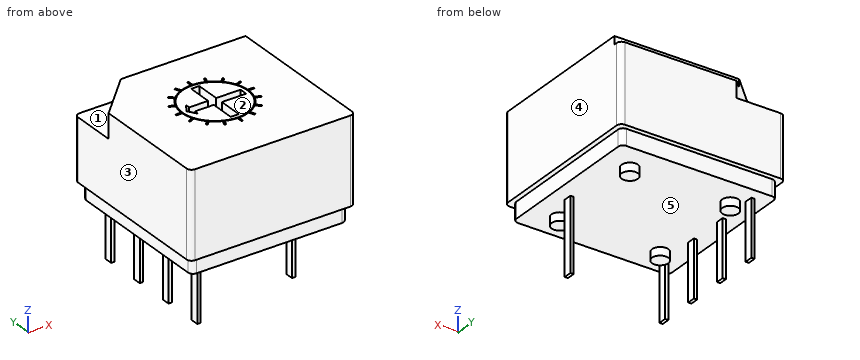
```python
from build123d import *

# Parameters (mm, degrees)
SKETCH1_W               = 10.2
SKETCH1_H               = 10.2
BOSS_EXTRUDE2_DEPTH     = 6.5
SKETCH3_R               = 0.501534086
BOSS_EXTRUDE3_DEPTH     = 0.5
FILLET1_R               = 0.3
SKETCH4_W               = 10.2
SKETCH4_H               = 10.2
SKETCH4_W_2             = 9.6
SKETCH4_H_2             = 9.6
CUT_EXTRUDE_THIN1_DEPTH = 1
FILLET2_R               = 0.3
SKETCH5_W               = 0.2
SKETCH5_H               = 0.5
BOSS_EXTRUDE5_DEPTH     = 3.5
SKETCH6_W               = 0.2
SKETCH6_H               = 0.5
BOSS_EXTRUDE6_DEPTH     = 1
SKETCH7_W               = 10.2
SKETCH7_H               = 10.2
CUT_EXTRUDE3_DEPTH      = 0.2
CUT_EXTRUDE4_DEPTH      = 1.5
CUT_EXTRUDE5_DEPTH      = 0.5
SKETCH10_R              = 2.05
SKETCH10_R_2            = 2
CUT_EXTRUDE6_DEPTH      = 0.5
CUT_EXTRUDE7_DEPTH      = 1
CUT_EXTRUDE8_DEPTH      = 0.3


with BuildPart() as part:
    # Sketch1 → Boss-Extrude2 (new body)
    with BuildSketch(Plane.XY):
        with Locations((5.1, 5.1)):
            Rectangle(SKETCH1_W, SKETCH1_H)
    extrude(amount=BOSS_EXTRUDE2_DEPTH)

    # Sketch3 → Boss-Extrude3 (add)
    with BuildSketch(Plane(origin=(0, 0, 0), x_dir=(-1, 0, 0), z_dir=(0, 0, -1))):
        with Locations((-8.2, 8.2)):
            Circle(SKETCH3_R)
        with Locations(Location((-2, 8.2, 0), (0, 0, 180))):
            Circle(SKETCH3_R)
        with Locations(Location((-8.2, 2, 0), (0, 0, 180))):
            Circle(SKETCH3_R)
        with Locations((-2, 2)):
            Circle(SKETCH3_R)
    extrude(amount=BOSS_EXTRUDE3_DEPTH)

    # Fillet1
    fillet1_edges = [part.edges().sort_by_distance(p)[0] for p in [
        (0, 10.2, 3.25),
        (10.2, 10.2, 3.25),
        (10.2, 0, 3.25),
        (0, 0, 3.25),
    ]]
    fillet(fillet1_edges, radius=FILLET1_R)

    # Sketch4 → Cut-Extrude-Thin1 (cut)
    with BuildSketch(Plane(origin=(0, 0, 0), x_dir=(-1, 0, 0), z_dir=(0, 0, -1))):
        with Locations((-5.1, 5.1)):
            Rectangle(SKETCH4_W, SKETCH4_H)
        with Locations((-5.1, 5.1)):
            Rectangle(SKETCH4_W_2, SKETCH4_H_2, mode=Mode.SUBTRACT)
    extrude(amount=-CUT_EXTRUDE_THIN1_DEPTH, mode=Mode.SUBTRACT)

    # Fillet2
    fillet2_edges = [part.edges().sort_by_distance(p)[0] for p in [
        (9.9, 0.3, 0.5),
        (9.9, 9.9, 0.5),
        (0.3, 9.9, 0.5),
        (0.3, 0.3, 0.5),
    ]]
    fillet(fillet2_edges, radius=FILLET2_R)

    # Sketch5 → Boss-Extrude5 (add)
    with BuildSketch(Plane(origin=(0, 0, 0), x_dir=(-1, 0, 0), z_dir=(0, 0, -1))):
        with Locations((-1.29, 8.935868973)):
            Rectangle(SKETCH5_W, SKETCH5_H)
        with Locations((-1.29, 6.395868973)):
            Rectangle(SKETCH5_W, SKETCH5_H)
        with Locations((-1.29, 3.855868973)):
            Rectangle(SKETCH5_W, SKETCH5_H)
        with Locations((-1.29, 1.315868973)):
            Rectangle(SKETCH5_W, SKETCH5_H)
        with Locations((-8.91, 3.855868973)):
            Rectangle(SKETCH5_W, SKETCH5_H)
    extrude(amount=BOSS_EXTRUDE5_DEPTH)

    # Sketch6 → Boss-Extrude6 (add)
    with BuildSketch(Plane(origin=(0, 0, -3.5), x_dir=(-1, 0, 0), z_dir=(0, 0, -1))):
        with Locations((-8.91, 3.855868973)):
            Rectangle(SKETCH6_W, SKETCH6_H)
    extrude(amount=BOSS_EXTRUDE6_DEPTH)

    # Sketch7 → Cut-Extrude3 (cut)
    with BuildSketch(Plane.XY.offset(6.5)):
        with Locations((5.1, 5.1)):
            Rectangle(SKETCH7_W, SKETCH7_H)
    extrude(amount=-CUT_EXTRUDE3_DEPTH, mode=Mode.SUBTRACT)

    # Sketch8 → Cut-Extrude4 (cut)
    with BuildSketch(Plane.XY.offset(6.3)):
        Polygon((0, 10.2), (0, 7.2), (3, 10.2), align=None)
    extrude(amount=-CUT_EXTRUDE4_DEPTH, mode=Mode.SUBTRACT)

    # Sketch9 → Cut-Extrude5 (cut)
    with BuildSketch(Plane.XY.offset(6.3)):
        Polygon((3, 10.2), (10.2, 10.2), (10.2, 9.7), (2.5, 9.7), align=None)
    extrude(amount=-CUT_EXTRUDE5_DEPTH, mode=Mode.SUBTRACT)

    # Sketch10 → Cut-Extrude6 (cut)
    with BuildSketch(Plane.XY.offset(6.3)):
        with Locations((5.1, 5.1)):
            Circle(SKETCH10_R)
        with Locations((5.1, 5.1)):
            Circle(SKETCH10_R_2, mode=Mode.SUBTRACT)
    extrude(amount=-CUT_EXTRUDE6_DEPTH, mode=Mode.SUBTRACT)

    # Sketch11 → Cut-Extrude7 (cut)
    with BuildSketch(Plane.XY.offset(6.3)):
        Polygon((5.35, 6.85), (5.35, 5.35), (6.85, 5.35), (6.85, 4.85), (5.35, 4.85), (5.35, 3.35), (4.85, 3.35), (4.85, 4.85), (3.683893811, 4.85), (3.683893811, 4.56171007), (3.35, 5.1), (3.683893811, 5.645083537), (3.683893811, 5.35), (4.85, 5.35), (4.85, 6.85), align=None)
    extrude(amount=-CUT_EXTRUDE7_DEPTH, mode=Mode.SUBTRACT)

    # Sketch12 → Cut-Extrude8 (cut)
    with BuildSketch(Plane.XY.offset(6.3)):
        with BuildLine():
            Line((5.05, 7.509113019), (5.15, 7.509113019))
            Line((5.15, 7.509113019), (5.15, 7.149390153))
            ThreePointArc((5.15, 7.149390153), (5.1, 7.15), (5.05, 7.149390153))
            Line((5.05, 7.149390153), (5.05, 7.509113019))
        make_face()
        with BuildLine():
            Line((4.224266338, 7.344864381), (4.131878384, 7.306596038))
            Line((4.131878384, 7.306596038), (4.269538365, 6.974255445))
            ThreePointArc((4.269538365, 6.974255445), (4.315498964, 6.993953042), (4.361926319, 7.012523788))
            Line((4.361926319, 7.012523788), (4.224266338, 7.344864381))
        make_face()
        with BuildLine():
            Line((2.855135619, 5.975733662), (3.187476212, 5.838073681))
            ThreePointArc((3.187476212, 5.838073681), (3.206046958, 5.884501036), (3.225744555, 5.930461635))
            Line((3.225744555, 5.930461635), (2.893403962, 6.068121616))
            Line((2.893403962, 6.068121616), (2.855135619, 5.975733662))
        make_face()
        with BuildLine():
            Line((2.690886981, 5.15), (2.690886981, 5.05))
            Line((2.690886981, 5.05), (3.050609847, 5.05))
            ThreePointArc((3.050609847, 5.05), (3.05, 5.1), (3.050609847, 5.15))
            Line((3.050609847, 5.15), (2.690886981, 5.15))
        make_face()
        with BuildLine():
            Line((3.431855187, 6.838855491), (3.361144509, 6.768144813))
            Line((3.361144509, 6.768144813), (3.615506986, 6.513782336))
            ThreePointArc((3.615506986, 6.513782336), (3.650431099, 6.549568901), (3.686217664, 6.584493014))
            Line((3.686217664, 6.584493014), (3.431855187, 6.838855491))
        make_face()
        with BuildLine():
            Line((3.431855187, 3.361144509), (3.686217664, 3.615506986))
            ThreePointArc((3.686217664, 3.615506986), (3.650431099, 3.650431099), (3.615506986, 3.686217664))
            Line((3.615506986, 3.686217664), (3.361144509, 3.431855187))
            Line((3.361144509, 3.431855187), (3.431855187, 3.361144509))
        make_face()
        with BuildLine():
            Line((4.131878384, 2.893403962), (4.224266338, 2.855135619))
            Line((4.224266338, 2.855135619), (4.361926319, 3.187476212))
            ThreePointArc((4.361926319, 3.187476212), (4.315498964, 3.206046958), (4.269538365, 3.225744555))
            Line((4.269538365, 3.225744555), (4.131878384, 2.893403962))
        make_face()
        with BuildLine():
            Line((5.15, 2.690886981), (5.15, 3.050609847))
            ThreePointArc((5.15, 3.050609847), (5.1, 3.05), (5.05, 3.050609847))
            Line((5.05, 3.050609847), (5.05, 2.690886981))
            Line((5.05, 2.690886981), (5.15, 2.690886981))
        make_face()
        with BuildLine():
            Line((6.068121616, 2.893403962), (5.930461635, 3.225744555))
            ThreePointArc((5.930461635, 3.225744555), (5.884501036, 3.206046958), (5.838073681, 3.187476212))
            Line((5.838073681, 3.187476212), (5.975733662, 2.855135619))
            Line((5.975733662, 2.855135619), (6.068121616, 2.893403962))
        make_face()
        with BuildLine():
            Line((6.768144813, 3.361144509), (6.838855491, 3.431855187))
            Line((6.838855491, 3.431855187), (6.584493014, 3.686217664))
            ThreePointArc((6.584493014, 3.686217664), (6.549568901, 3.650431099), (6.513782336, 3.615506986))
            Line((6.513782336, 3.615506986), (6.768144813, 3.361144509))
        make_face()
        with BuildLine():
            Line((2.855135619, 4.224266338), (2.893403962, 4.131878384))
            Line((2.893403962, 4.131878384), (3.225744555, 4.269538365))
            ThreePointArc((3.225744555, 4.269538365), (3.206046958, 4.315498964), (3.187476212, 4.361926319))
            Line((3.187476212, 4.361926319), (2.855135619, 4.224266338))
        make_face()
        with BuildLine():
            Line((7.344864381, 4.224266338), (7.012523788, 4.361926319))
            ThreePointArc((7.012523788, 4.361926319), (6.993953042, 4.315498964), (6.974255445, 4.269538365))
            Line((6.974255445, 4.269538365), (7.306596038, 4.131878384))
            Line((7.306596038, 4.131878384), (7.344864381, 4.224266338))
        make_face()
        with BuildLine():
            Line((7.509113019, 5.15), (7.149390153, 5.15))
            ThreePointArc((7.149390153, 5.15), (7.15, 5.1), (7.149390153, 5.05))
            Line((7.149390153, 5.05), (7.509113019, 5.05))
            Line((7.509113019, 5.05), (7.509113019, 5.15))
        make_face()
        with BuildLine():
            Line((7.344864381, 5.975733662), (7.306596038, 6.068121616))
            Line((7.306596038, 6.068121616), (6.974255445, 5.930461635))
            ThreePointArc((6.974255445, 5.930461635), (6.993953042, 5.884501036), (7.012523788, 5.838073681))
            Line((7.012523788, 5.838073681), (7.344864381, 5.975733662))
        make_face()
        with BuildLine():
            Line((6.768144813, 6.838855491), (6.513782336, 6.584493014))
            ThreePointArc((6.513782336, 6.584493014), (6.549568901, 6.549568901), (6.584493014, 6.513782336))
            Line((6.584493014, 6.513782336), (6.838855491, 6.768144813))
            Line((6.838855491, 6.768144813), (6.768144813, 6.838855491))
        make_face()
        with BuildLine():
            Line((5.975733662, 7.344864381), (5.838073681, 7.012523788))
            ThreePointArc((5.838073681, 7.012523788), (5.884501036, 6.993953042), (5.930461635, 6.974255445))
            Line((5.930461635, 6.974255445), (6.068121616, 7.306596038))
            Line((6.068121616, 7.306596038), (5.975733662, 7.344864381))
        make_face()
    extrude(amount=-CUT_EXTRUDE8_DEPTH, mode=Mode.SUBTRACT)


solid = part.part
```
The listing builds one solid part. Answer for the finished solid, in the listing's coordinates (mm). Face numbers are marked on the shaded views. A direction names the side the tool comes from. Coordinates: 2 decimals unless noted, no trailing zeros. Loops run counter-clockwise (first coordinate to the right, second up) from the corner with the lowest first, then second, coordinate; pieces in that order, holes last. Notation, with made-up numbers: (31, 16) -> (53, 16) arc R13 ccw to (53, 33) -> close; hole circle Ø5 at (-30, 53). An arc over 180 degrees is marked (long way). Return JSON: item names as keys, results as strings. Group by question number.
(1) Find the intervals of material crossed by probe 1 along Y at (x, z) = (5.1, 6.1); probe 2 along X at (y, z) = (3.75, 5.75); probe 3 along Z at (x, y) = (2.5, 1.5), in increasing order. Write a range as from..to.
(2) A cutting plane is placed at B-B on x = 2. Write down the section's boundary in (y, z), and give its area (3 significant figures).
(3) Given pin 1 Ø2 at (x, y) = (5.5, 6) entering from -Z; pin 2 Ø0.8 at (y, z) = (3, 0.5) entering from -X; pin 3 Ø0.5 at (y, z) = (4, -1.5) entering from +X, each flat-ended and moving along its own axis, determine where each tip first touches the part or whether it passes through.
(4) A cutting plane is placed at C-C on y = 2. Write down the section's boundary in (x, z).
(5) Which of the six approach directions +Z, -Z, +X, -X, +Y, -Y give full straight-line access (tool end or side, diameter ignored) to the marked faces 1 and 2?
(6) Determine the mould class of the marked faces 3, 4 and 5 for opening direction X: released by +X, released by -X, zero draft, split by the parting line, or undercut.
(7) A cutting plane is placed at A-A on z = -0.75. Write down the section's boundary in (x, y), and give its area (3 significant figures).
(8) A cutting plane is placed at D-D on y = 8.2. Write down the section's boundary in (x, z).
The answers:
{
 "1": {"probe 1": "y = 0..2.69, 3.1..3.35, 6.85..7.1, 7.51..9.7", "probe 2": "x = 0..4.85, 5.35..10.2", "probe 3": "z = 0..6.3"},
 "2": {"outline": "(0, 1) -> (0.3, 1) -> (0.3, 0) -> (1.5, 0) -> (1.5, -0.5) -> (2.5, -0.5) -> (2.5, 0) -> (7.7, 0) -> (7.7, -0.5) -> (8.7, -0.5) -> (8.7, 0) -> (9.9, 0) -> (9.9, 1) -> (10.2, 1) -> (10.2, 4.8) -> (9.2, 4.8) -> (9.2, 6.3) -> (0, 6.3) -> close", "area": "63.2 mm^2"},
 "3": {"pin 1": "stops at z = 0", "pin 2": "stops at x = 0.3", "pin 3": "stops at x = 9.01"},
 "4": {"outline": "(0, 1) -> (0.3, 1) -> (0.3, 0) -> (1.5, 0) -> (1.5, -0.5) -> (2.5, -0.5) -> (2.5, 0) -> (7.7, 0) -> (7.7, -0.5) -> (8.7, -0.5) -> (8.7, 0) -> (9.9, 0) -> (9.9, 1) -> (10.2, 1) -> (10.2, 6.3) -> (0, 6.3) -> close"},
 "5": {"face 1": "+Z, -X, +Y", "face 2": "+Z, +X, -X, +Y, -Y"},
 "6": {"face 3": "released by -X", "face 4": "released by +X", "face 5": "undercut"},
 "7": {"outline": "(1.19, 1.07) -> (1.39, 1.07) -> (1.39, 1.57) -> (1.19, 1.57) -> close; (1.19, 3.61) -> (1.39, 3.61) -> (1.39, 4.11) -> (1.19, 4.11) -> close; (1.19, 6.15) -> (1.39, 6.15) -> (1.39, 6.65) -> (1.19, 6.65) -> close; (1.19, 8.69) -> (1.39, 8.69) -> (1.39, 9.19) -> (1.19, 9.19) -> close; (8.81, 3.61) -> (9.01, 3.61) -> (9.01, 4.11) -> (8.81, 4.11) -> close", "area": "0.500 mm^2"},
 "8": {"outline": "(0, 1) -> (0.3, 1) -> (0.3, 0) -> (1.5, 0) -> (1.5, -0.5) -> (2.5, -0.5) -> (2.5, 0) -> (7.7, 0) -> (7.7, -0.5) -> (8.7, -0.5) -> (8.7, 0) -> (9.9, 0) -> (9.9, 1) -> (10.2, 1) -> (10.2, 6.3) -> (1, 6.3) -> (1, 4.8) -> (0, 4.8) -> close"}
}
